Design review of the part shown in the three views and the two pictorial views. Dimensions are in mm from the part's minimum x, y and z. A direction names the side the tool comes from. Coordinates: 2 decimals unless noted, no trailing zeros. Loops run counter-clockwise (first coordinate to the right, second up) from the corner with the lowest first, then second, coordinate; pieces in that order, holes last. Notation, with made-up numbers: (-1.75, -38.75) - (19.25, -38.75) arc R34 cw to (19.25, -0.75) - close; hole circle Ø7 at (64.25, -28). An arc over 180 degrees is marked (long way). One line per item, written item: value. Start each with the question number.
1. Take a section at A-A, the plane x = 66. State the section outline as (y, z) points, and give its area (3 significant figures).
2. Insertion check: pin 1 (8 mm diameter, centred on y = 19.5, z = 5.5, fed in from +X); pin 2 (8 mm diameter, centred on y = 28.5, z = 16.5, fed in from -X); pin 3 (15 mm diameter, centred on x = 48, z = 14.5, fed in from +Y). Each pin has a flat end and moves straight along its axis. Give the tip position at first contact, or say it passes through.
3. Take a section at B-B, the plane y = 25. State the section outline as (x, z) points, and give its area (3 significant figures).
4. To check wall thickness, follow line 1 (X direction, y = 10, z = 22); line 2 (Y direction, x = 40.5, z = 12). State the ranges of each line that lie inside material, in increasing order. Write a range as from..to.
5. Take a section at C-C, the plane z = 3.5. State the section outline as (x, y) points, and give its area (3 significant figures).
6. For the marked faces 1, 2, 3 and 4, list the 3-axis set-ups (+Z, -Z, +X, -X, +Y, -Y) from which the entire face can be reached by the end or side of a thin tool; tool diameter is ignored.
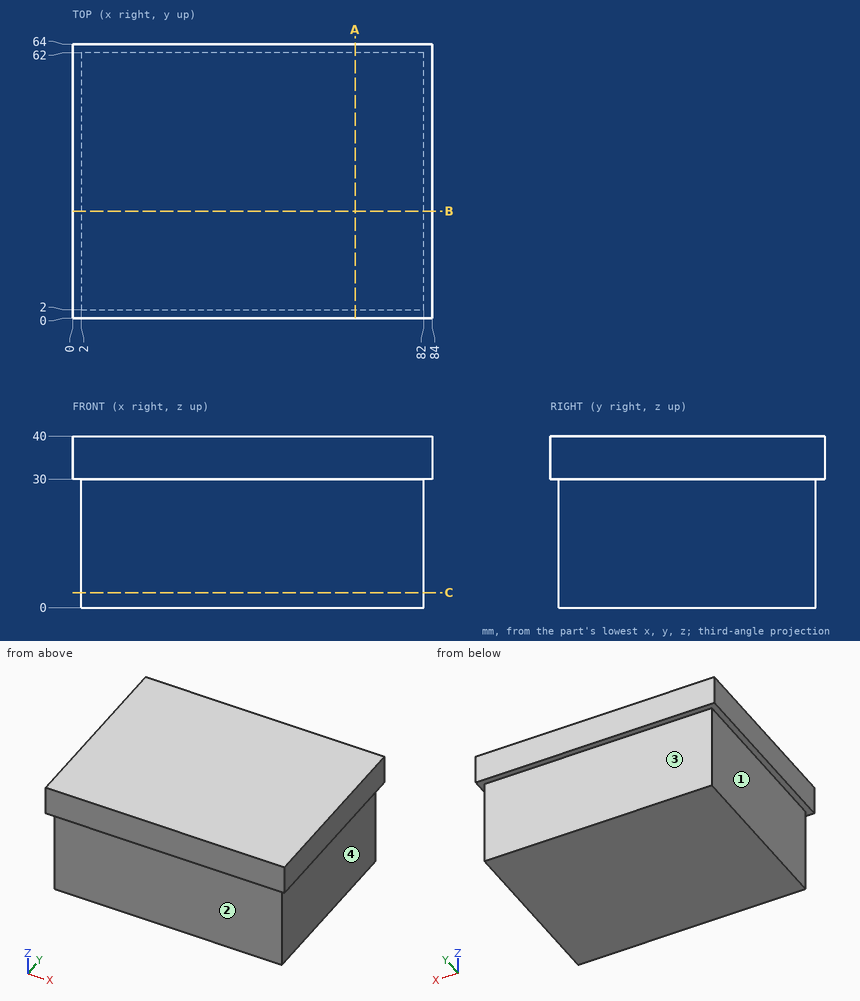
Solutions:
1. outline: (0, 30) - (2, 30) - (2, 0) - (62, 0) - (62, 30) - (64, 30) - (64, 40) - (0, 40) - close
1. area: 2,440 mm2
2. pin 1: x = 82
2. pin 2: x = 2
2. pin 3: y = 62
3. outline: (0, 30) - (2, 30) - (2, 0) - (82, 0) - (82, 30) - (84, 30) - (84, 40) - (0, 40) - close
3. area: 3,240 mm2
4. line 1: 2..82
4. line 2: 2..62
5. outline: (2, 2) - (82, 2) - (82, 62) - (2, 62) - close
5. area: 4,800 mm2
6. face 1: -Z, -X, +Y, -Y
6. face 2: -Z, +X, -X, -Y
6. face 3: -Z, +X, -X, +Y
6. face 4: -Z, +X, +Y, -Y
